Geometry check sheet. Reference: the model listing, model coordinates, mm. Face numbers are marked on the shaded views. A direction names the side the tool comes from. Coordinates: 2 decimals unless noted, no trailing zeros. Write each loop counter-clockwise with the first axis right and the second up, starting at its lowest first coordinate (ties: lowest second). Pieces come first, ordered by that corner, then holes. Notation, with made-up numbers: (47.25, 55.25) -> (73.25, 55.25) arc R18 cw to (73.25, 67.25) -> close; hole circle Ø7 at (32, 18.25). An arc over 180 degrees is marked (long way). Answer in a Markdown table with one row per item. Add a question column.
1. Mould release check, pull along X, two halves, no side actions. Record for the marked faces 4, 5, 6 and 7: pulls with the +X half, pulls with the -X half, needs draft (parallel to the pull), parting line crosses it, or undercut.
2. Cross-section at A-A on z = 3.3. Give the number of separate pieces and of enclosed holes in the cut face, and give its area (3 significant figures).
3. Scan lines: L1, parallel to Y at x = -18, z = 3.2; L2, parallel to Y at x = -15, z = 3.75; L3, parallel to X at y = -0.5, z = 2.6. Record each from-to range of solid material in increasing order. Write a range as from..to.
4. Cross-section at B-B on x = -7. Record the cut outline in (y, z).
5. Depth check by flat-ended pin: P1, Ø1.2, axis at x = -5.5, z = 1.5, coming from the +Y side; P2, Ø6.5, axis at x = 15.22, y = 0, coming from the +Z side; P3, Ø2, axis at x = -8, z = 3, coming from the -Y side. Enter the tip coordinate at first touch or a pass-through.
6. Set-up check for the marked faces 1, 2 and 3: record each of +Z, -Z, +X, -X, +Y, -Y from which the full face is reachable in a straight line by a thin tool's end or side.
```python
from build123d import *

# Parameters (mm, degrees)
SKETCH1_R           = 1.5
BOSS_EXTRUDE1_DEPTH = 4
CUT_EXTRUDE1_DEPTH  = 23.415528994
CIRPATTERN1_COUNT   = 12
SKETCH3_W           = 11.336678395
SKETCH3_H           = 5
BOSS_EXTRUDE2_DEPTH = 4
SKETCH4_R           = 2.5
CUT_EXTRUDE2_DEPTH  = 23.415528994


with BuildPart() as part:
    # Sketch1 → Boss-Extrude1 (new body)
    with BuildSketch(Plane.XY):
        with BuildLine():
            Line((-18, 2.5), (9.769591268, 2.5))
            ThreePointArc((9.769591268, 2.5), (21.223947325, 0), (9.769591268, -2.5))
            Line((9.769591268, -2.5), (-18, -2.5))
            ThreePointArc((-18, -2.5), (-20.5, 0), (-18, 2.5))
        make_face()
        with Locations((-18, 0)):
            Circle(SKETCH1_R, mode=Mode.SUBTRACT)
    extrude(amount=BOSS_EXTRUDE1_DEPTH)

    # Sketch2 → Cut-Extrude1 (cut, through all)
    with BuildSketch(Plane.XY.offset(4)):
        with BuildLine():
            Line((15.878876805, 4.81), (15.943947325, 5.06))
            ThreePointArc((15.943947325, 5.06), (15.813826986, 5.706078038), (15.223947325, 6))
            ThreePointArc((15.223947325, 6), (16.816567466, 5.943739283), (18.223947325, 5.196152423))
            ThreePointArc((18.223947325, 5.196152423), (17.566135573, 5.236548367), (17.130409034, 4.742088543))
            Line((17.130409034, 4.742088543), (17.061761758, 4.493046932))
            ThreePointArc((17.061761758, 4.493046932), (16.312974518, 4.064304815), (15.878876805, 4.81))
        make_face()
    cut_extrude1 = extrude(amount=-CUT_EXTRUDE1_DEPTH, mode=Mode.SUBTRACT)

    # CirPattern1: Cut-Extrude1 ×12 about axis
    cirpattern1_axis = Axis((15.223947325, 0, 0), (0, 0, 1))
    for i in range(1, CIRPATTERN1_COUNT):
        add(cut_extrude1.rotate(cirpattern1_axis, i * 360 / CIRPATTERN1_COUNT), mode=Mode.SUBTRACT)

    # Sketch3 → Boss-Extrude2 (add)
    with BuildSketch(Plane.XY.offset(4)):
        with Locations((11.656973093, 0)):
            Rectangle(SKETCH3_W, SKETCH3_H)
    extrude(amount=-BOSS_EXTRUDE2_DEPTH)

    # Sketch4 → Cut-Extrude2 (cut, through all)
    with BuildSketch(Plane.XY.offset(4)):
        with Locations((15.223947325, 0)):
            Circle(SKETCH4_R)
    extrude(amount=-CUT_EXTRUDE2_DEPTH, mode=Mode.SUBTRACT)


solid = part.part
```
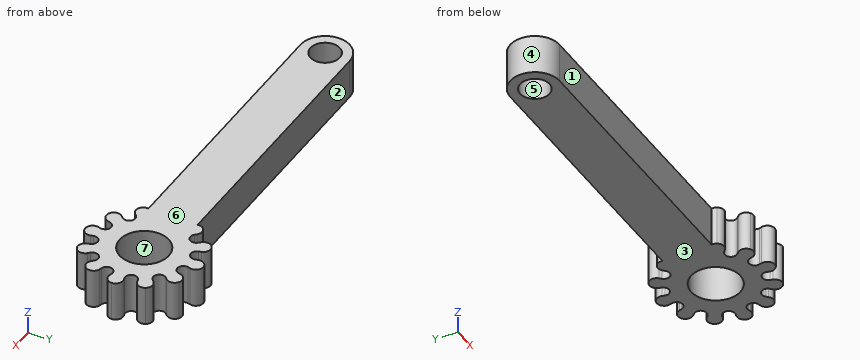
Results found:
| question | item | result |
|---|---|---|
| 1 | face 4 | pulls with the -X half |
| 1 | face 5 | undercut |
| 1 | face 6 | needs draft |
| 1 | face 7 | undercut |
| 2 | separate pieces | 1 |
| 2 | enclosed holes | 2 |
| 2 | area | 209 mm^2 |
| 3 | L1 | y = -2.5..-1.5, 1.5..2.5 |
| 3 | L2 | y = -2.5..2.5 |
| 3 | L3 | x = -20.45..-19.41, -16.59..12.77, 17.67..21.03 |
| 4 | outline | (-2.5, 0) -> (2.5, 0) -> (2.5, 4) -> (-2.5, 4) -> close |
| 5 | P1 | stops at y = 2.5 |
| 5 | P2 | stops at z = 4 |
| 5 | P3 | stops at y = -2.5 |
| 6 | face 1 | +Z, -Z, -X, -Y |
| 6 | face 2 | +Z, -Z, -X, +Y |
| 6 | face 3 | -Z, +X, -X, +Y, -Y |
